For this review, take the finished solid that the model builds, in its own axes (mm). A direction names the side the tool comes from. Round coordinates to 2 decimals unless told otherwise and drop trailing zeros. Order: outer loops, then holes, each group sorted by start corner. A loop starts at its lowest first (then second) coordinate and runs counter-clockwise, first axis right, second up. Notation, with made-up numbers: M 62.25,23.25 L 113.25,23.25 A24 ccw 113.25,54.25 Z; hole C -15,-4.75 d9. An arc over 180 degrees is marked long. Answer as a JSON object with one key per item and string values.
from build123d import *

# Parameters (mm, degrees)
SKETCH1_W             = 3.175
SKETCH1_H             = 12.7
BOSS_EXTRUDE1_DEPTH   = 6.35
SKETCH1_W_2           = 11.11
BOSS_EXTRUDE1_2_DEPTH = 6.35
BOSS_EXTRUDE1_3_DEPTH = 6.35
BOSS_EXTRUDE1_4_DEPTH = 6.35
SKETCH1_W_3           = 1.595
BOSS_EXTRUDE1_5_DEPTH = 6.35
SKETCH1_3_W           = 6.35
SKETCH1_3_H           = 12.7
BOSS_EXTRUDE2_DEPTH   = 12.7
SKETCH3_W             = 63.5
SKETCH3_H             = 12.7
BOSS_EXTRUDE3_DEPTH   = 38.1
CUT_EXTRUDE1_DEPTH    = 75.324844433
SKETCH5_W             = 50.8
SKETCH5_H             = 22.225
CUT_EXTRUDE2_DEPTH    = 44.273418952
FILLET1_R             = 2.54


with BuildPart() as part:
    # Sketch1 → Boss-Extrude1 (new body)
    with BuildSketch(Plane(origin=(0, 0, 0), x_dir=(1, 0, 0), z_dir=(0, 1, 0))):
        with Locations((-30.1625, 0)):
            Rectangle(SKETCH1_W, SKETCH1_H)
    extrude(amount=BOSS_EXTRUDE1_DEPTH)



with BuildPart() as body_2:
    # Sketch1 → Boss-Extrude1 2 (new body)
    with BuildSketch(Plane(origin=(0, 0, 0), x_dir=(1, 0, 0), z_dir=(0, 1, 0))):
        with Locations((-16.67, 0)):
            Rectangle(SKETCH1_W_2, SKETCH1_H)
    extrude(amount=BOSS_EXTRUDE1_2_DEPTH)


with BuildPart() as body_3:
    # Sketch1 → Boss-Extrude1 3 (new body)
    with BuildSketch(Plane(origin=(0, 0, 0), x_dir=(1, 0, 0), z_dir=(0, 1, 0))):
        with Locations((0.79, 0)):
            Rectangle(SKETCH1_W_2, SKETCH1_H)
    extrude(amount=BOSS_EXTRUDE1_3_DEPTH)


with BuildPart() as body_4:
    # Sketch1 → Boss-Extrude1 4 (new body)
    with BuildSketch(Plane(origin=(0, 0, 0), x_dir=(1, 0, 0), z_dir=(0, 1, 0))):
        with Locations((18.25, 0)):
            Rectangle(SKETCH1_W_2, SKETCH1_H)
    extrude(amount=BOSS_EXTRUDE1_4_DEPTH)


with BuildPart() as body_5:
    # Sketch1 → Boss-Extrude1 5 (new body)
    with BuildSketch(Plane(origin=(0, 0, 0), x_dir=(1, 0, 0), z_dir=(0, 1, 0))):
        with Locations((30.9525, 0)):
            Rectangle(SKETCH1_W_3, SKETCH1_H)
    extrude(amount=BOSS_EXTRUDE1_5_DEPTH)


with BuildPart() as part_1:
    add(part.part)

    add(body_2.part)  # Boss-Extrude2 merges body 2

    add(body_3.part)  # Boss-Extrude2 merges body 3

    add(body_4.part)  # Boss-Extrude2 merges body 4

    add(body_5.part)  # Boss-Extrude2 merges body 5
    # Sketch1_3 → Boss-Extrude2 (add)
    with BuildSketch(Plane(origin=(0, 0, 0), x_dir=(1, 0, 0), z_dir=(0, 1, 0))):
        with Locations((-25.4, 0)):
            Rectangle(SKETCH1_3_W, SKETCH1_3_H)
        with Locations((-7.94, 0)):
            Rectangle(SKETCH1_3_W, SKETCH1_3_H)
        with Locations((9.52, 0)):
            Rectangle(SKETCH1_3_W, SKETCH1_3_H)
        with Locations((26.98, 0)):
            Rectangle(SKETCH1_3_W, SKETCH1_3_H)
    extrude(amount=BOSS_EXTRUDE2_DEPTH)

    # Sketch3 → Boss-Extrude3 (add)
    with BuildSketch(Plane(origin=(0, 0, 0), x_dir=(-1, 0, 0), z_dir=(0, -1, 0))):
        Rectangle(SKETCH3_W, SKETCH3_H)
    extrude(amount=BOSS_EXTRUDE3_DEPTH)

    # Sketch4 → Cut-Extrude1 (cut, through all)
    with BuildSketch(Plane(origin=(31.75, 0, 0), x_dir=(0, 0, -1), z_dir=(1, 0, 0))):
        with BuildLine():
            Line((6.35, -26.518602675), (6.35, -38.1))
            Line((6.35, -38.1), (-6.35, -38.1))
            Line((-6.35, -38.1), (-6.35, -26.518602675))
            ThreePointArc((-6.35, -26.518602675), (0, -24.892), (6.35, -26.518602675))
        make_face()
    extrude(amount=-CUT_EXTRUDE1_DEPTH, mode=Mode.SUBTRACT)

    # Sketch5 → Cut-Extrude2 (cut, through all)
    with BuildSketch(Plane.XY.offset(6.35)):
        with Locations((0, -10.084301337)):
            Rectangle(SKETCH5_W, SKETCH5_H)
    extrude(amount=-CUT_EXTRUDE2_DEPTH, mode=Mode.SUBTRACT)

    # Fillet1
    fillet1_edges = [part_1.edges().sort_by_distance(p)[0] for p in [
        (0, -21.196801337, -6.35),
        (25.4, -10.084301337, -6.35),
        (0, 1.028198663, -6.35),
        (-25.4, -10.084301337, -6.35),
        (-25.4, -21.196801337, 0),
        (-25.4, 1.028198663, 0),
        (25.4, 1.028198663, 0),
        (25.4, -21.196801337, 0),
        (-25.4, -10.084301337, 6.35),
        (0, -21.196801337, 6.35),
        (25.4, -10.084301337, 6.35),
        (0, 1.028198663, 6.35),
    ]]
    fillet(fillet1_edges, radius=FILLET1_R)


solid = part_1.part
1) Machinability: for faces 4 (the cylindrical face through (24.68, -20.43, -0.05)), 5 (the cylindrical face through (0.32, -21.961, 5.626)), 6 (the flat face through (-4.765, 9, 0)), 7 (the cylindrical face through (26.164, -10.204, -5.626)), which of the approach directions +Z, -Z, +X, -X, +Y, -Y give a long, thin tool a straight path to every point of the face, cutting with its end or side? Answer none if there is none.
Geometry check:
{"face 4": "+Z, -Z", "face 5": "+Z", "face 6": "+Z, -Z, +Y", "face 7": "-Z"}
2) Insertion check: P1, Ø4, axis at x = -11, z = -1, coming from the -Y side; P2, Ø1.9, axis at y = 9.5, z = -0.5, coming from the -X side (3 decimals); P3, Ø7, axis at y = 11, z = 0, coming from the +X side (3 decimals). Each pin has a flat end and moves straight along its axis. Give the tip position at first contact, or say it passes through.
Geometry check:
{"P1": "stops at y = -25.24", "P2": "stops at x = -28.575", "P3": "stops at x = 30.155"}
3) Add section A-A on x = -9. State the section outline as (y, z) points.
Geometry check:
{"outline": "M -26.52,-6.35 L -23.74,-6.35 A2.54 ccw -21.2,-3.81 L -21.2,3.81 A2.54 ccw -23.74,6.35 L -26.52,6.35 A13.21 cw Z; M 1.03,-3.81 A2.54 ccw 3.57,-6.35 L 12.7,-6.35 L 12.7,6.35 L 3.57,6.35 A2.54 ccw 1.03,3.81 Z"}
4) Add section C-C on y = -14.5. State the section outline as (x, z) points.
Geometry check:
{"outline": "M -31.75,-6.35 L -27.94,-6.35 A2.54 ccw -25.4,-3.81 L -25.4,3.81 A2.54 ccw -27.94,6.35 L -31.75,6.35 Z; M 25.4,-3.81 A2.54 ccw 27.94,-6.35 L 31.75,-6.35 L 31.75,6.35 L 27.94,6.35 A2.54 ccw 25.4,3.81 Z"}
5) Add section B-B on y = 10.5. State the section outline as (x, z) points (3 decimals), and give its area (3 significant figures).
Geometry check:
{"outline": "M -28.575,-6.35 L -22.225,-6.35 L -22.225,6.35 L -28.575,6.35 Z; M -11.115,-6.35 L -4.765,-6.35 L -4.765,6.35 L -11.115,6.35 Z; M 6.345,-6.35 L 12.695,-6.35 L 12.695,6.35 L 6.345,6.35 Z; M 23.805,-6.35 L 30.155,-6.35 L 30.155,6.35 L 23.805,6.35 Z", "area": "323 mm²"}
6) Mouldability with a two-part tool opening along X and no side actions: class faces 1 (the flat face through (-28.575, 9, 0)), 2 (the flat face through (0, 5, 6.35)), 3 (the cylindrical face through (0.32, 1.792, 5.626)) as +X half, -X half, draft (parallel to the pull), parting line (faces both ways), or undercut.
Geometry check:
{"face 1": "-X half", "face 2": "draft", "face 3": "undercut"}
7) For L1, parallel to X at y = -9.5, z = -1.75; L2, parallel to X at y = 8, z = -3 (3 decimals); L3, parallel to Y at x = 17, z = 0.5, list the stretches that pass through material, from the lowest coordinate up.
Geometry check:
{"L1": "x = -31.75 to -25.4, 25.4 to 31.75", "L2": "x = -28.575 to -22.225, -11.115 to -4.765, 6.345 to 12.695, 23.805 to 30.155", "L3": "y = -24.9 to -21.2, 1.03 to 6.35"}
8) Add section D-D on z = -2.75. State the section outline as (x, y) points (3 decimals).
Geometry check:
{"outline": "M -31.75,-25.181 L 31.75,-25.181 L 31.75,6.35 L 30.155,6.35 L 30.155,12.7 L 23.805,12.7 L 23.805,6.35 L 12.695,6.35 L 12.695,12.7 L 6.345,12.7 L 6.345,6.35 L -4.765,6.35 L -4.765,12.7 L -11.115,12.7 L -11.115,6.35 L -22.225,6.35 L -22.225,12.7 L -28.575,12.7 L -28.575,6.35 L -31.75,6.35 Z; hole M -25.4,-18.657 A2.54 ccw -22.86,-21.197 L 22.86,-21.197 A2.54 ccw 25.4,-18.657 L 25.4,-1.512 A2.54 ccw 22.86,1.028 L -22.86,1.028 A2.54 ccw -25.4,-1.512 Z"}
